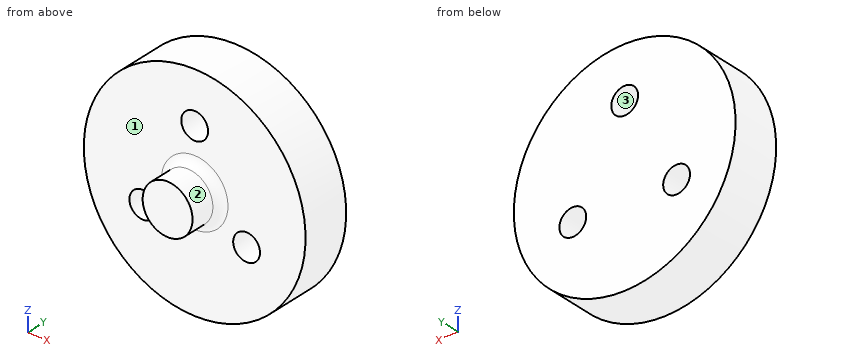
from build123d import *

# Parameters (mm, degrees)
SKETCH4_R           = 33.3
BOSS_EXTRUDE2_DEPTH = 15
SKETCH5_R           = 4.025
CUT_EXTRUDE1_DEPTH  = 50.424487858
SKETCH6_R           = 7.5
BOSS_EXTRUDE3_DEPTH = 10
FILLET1_R           = 2.5


with BuildPart() as part:
    # Sketch4 → Boss-Extrude2 (new body)
    with BuildSketch(Plane(origin=(0, 0, 0), x_dir=(1, 0, 0), z_dir=(0, 1, 0))):
        with Locations(Location((0, 0, 0), (0, 0, 270))):
            Circle(SKETCH4_R)
    extrude(amount=BOSS_EXTRUDE2_DEPTH)

    # Sketch5 → Cut-Extrude1 (cut, through all)
    with BuildSketch(Plane.XZ):
        with Locations(Location((0, 18, 0), (0, 0, 270))):
            Circle(SKETCH5_R)
        with Locations(Location((15.588457268, -9, 0), (0, 0, 270))):
            Circle(SKETCH5_R)
        with Locations(Location((-15.588457268, -9, 0), (0, 0, 270))):
            Circle(SKETCH5_R)
    extrude(amount=-CUT_EXTRUDE1_DEPTH, mode=Mode.SUBTRACT)

    # Sketch6 → Boss-Extrude3 (add)
    with BuildSketch(Plane.XZ):
        with Locations(Location((0, 0, 0), (0, 0, 90))):
            Circle(SKETCH6_R)
    extrude(amount=BOSS_EXTRUDE3_DEPTH)

    # Fillet1
    fillet1_edges = [part.edges().sort_by_distance(p)[0] for p in [
        (0, 0, -7.5),
    ]]
    fillet(fillet1_edges, radius=FILLET1_R)


solid = part.part
Read the model definition and answer for the solid it produces. Units are mm, in the model's axes. Face numbers are marked on the shaded views. Round coordinates to 2 decimals unless told otherwise and drop trailing zeros. Write each loop counter-clockwise with the first axis right and the second up, starting at its lowest first coordinate (ties: lowest second). Pieces come first, ordered by that corner, then holes. Notation, with made-up numbers: M 64,46.25 L 105,46.25 A32 ccw 105,74.25 Z; hole C 81.5,-1.5 d6. An arc over 180 degrees is marked long. Use a Markdown table: item, result.
1) Flat-ended cylindrical pins translate along their axes: pin 1 (10.5 mm diameter, centred on x = -15.59, z = -9, fed in from -Y); pin 2 (8 mm diameter, centred on x = -4.5, y = 3, fed in from +Z); pin 3 (1.5 mm diameter, centred on x = -16.5, y = 2.5, fed in from +Z); pin 4 (1.5 mm diameter, centred on y = -2, z = -19, fed in from -X). Find the tip coordinate at first contact, or state that the pin passes through.
Answers follow:
| item | result |
|---|---|
| pin 1 | stops at y = 0 |
| pin 2 | stops at z = 33.3 |
| pin 3 | stops at z = 29.34 |
| pin 4 | passes through |
2) The part is cut by section B-B (z = 0). Write down the section's boundary in (x, y).
Answers follow:
| item | result |
|---|---|
| outline | M -33.3,0 L -10,0 A2.5 cw -7.5,-2.5 L -7.5,-10 L 7.5,-10 L 7.5,-2.5 A2.5 cw 10,0 L 33.3,0 L 33.3,15 L -33.3,15 Z |
3) For a pull along X with two mould halves and no side action, classify the marked faces 1, 2 and 3 as pulls with the +X half, pulls with the -X half, needs draft (parallel to the pull), parting line crosses it, or undercut.
Answers follow:
| item | result |
|---|---|
| face 1 | needs draft |
| face 2 | parting line crosses it |
| face 3 | undercut |
4) The part is cut by section D-D (y = 13). Write down the section's boundary in (x, z) (3 decimals).
Answers follow:
| item | result |
|---|---|
| outline | C 0,0 d66.6; hole C -15.588,-9 d8.05; hole C 0,18 d8.05; hole C 15.588,-9 d8.05 |
5) The part is cut by section C-C (z = 18). Write down the section's boundary in (x, y) (3 decimals), plus the area to 3 significant figures.
Answers follow:
| item | result |
|---|---|
| outline | M -28.016,0 L -4.025,0 L -4.025,15 L -28.016,15 Z; M 4.025,0 L 28.016,0 L 28.016,15 L 4.025,15 Z |
| area | 720 mm2 |
6) The part is cut by section A-A (x = 0). Write down the section's boundary in (y, z) (3 decimals), plus the area to 3 significant figures.
Answers follow:
| item | result |
|---|---|
| outline | M -10,-7.5 L -2.5,-7.5 A2.5 cw 0,-10 L 0,-33.3 L 15,-33.3 L 15,13.975 L 0,13.975 L 0,10 A2.5 cw -2.5,7.5 L -10,7.5 Z; M 0,22.025 L 15,22.025 L 15,33.3 L 0,33.3 Z |
| area | 1,030 mm2 |
7) Straight lines are drawn through the part: line 1 along X through (y, z) = (4.25, -9); line 2 along Y through (x, z) = (30, -4); line 3 along Z through (x, y) = (-14, 4.5). For each, find the intervals that lie inside material, in ascending order. Write a range as [from, to].
Answers follow:
| item | result |
|---|---|
| line 1 | x = [-32.06, -19.61], [-11.56, 11.56], [19.61, 32.06] |
| line 2 | y = [0, 15] |
| line 3 | z = [-30.21, -12.7], [-5.3, 30.21] |
